Design review of the part shown in the three views and the two pictorial views. Dimensions are in mm from the part's minimum x, y and z. Round coordinates to 2 decimals unless told otherwise and drop trailing zeros. Loops run counter-clockwise (first coordinate to the right, second up) from the corner with the lowest first, then second, coordinate; pieces in that order, holes last. Notation, with made-up numbers: (77.5, -28.5) -> (130.5, -28.5) arc R21 ccw to (130.5, -6.5) -> close; hole circle Ø2 at (0, -31.75). An arc over 180 degrees is marked (long way). Write each question's results on one line, items separated by ' | '. Start each with the question number.
Item 1: We need section A-A (y = 22.5). Give the boundary of the cut face in (x, z) (3 decimals), and give its area (3 significant figures).
Item 2: Clearance check with flat-ended pins moving along their axes: pin 1 Ø10 at (x, y) = (51.5, 32) entering from -Z; pin 2 Ø8 at (x, y) = (35.875, 22.5) entering from +Z. State where each tip first meets the part, or that it passes through.
Item 3: We need section B-B (x = 37). Give the boundary of the cut face in (y, z).
Item 4: For L1, parallel to X at y = 22, z = 6.5; L2, parallel to Y at x = 37.5, z = 0.5; L3, parallel to Y at x = 130, z = 8.5, list the stretches that pass through material, from the lowest coordinate up. Write a range as from..to.
Item 5: We need section C-C (z = 2.5). Give the boundary of the cut face in (x, y) (3 decimals).
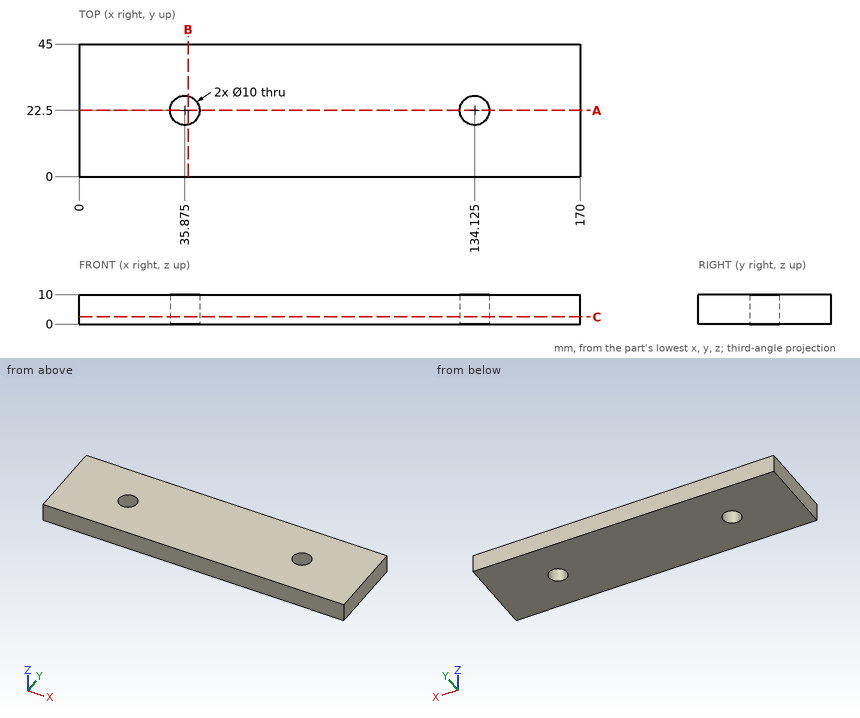
Here are the results:
1) outline: (0, 0) -> (30.875, 0) -> (30.875, 10) -> (0, 10) -> close; (40.875, 0) -> (129.125, 0) -> (129.125, 10) -> (40.875, 10) -> close; (139.125, 0) -> (170, 0) -> (170, 10) -> (139.125, 10) -> close | area: 1,500 mm2
2) pin 1: stops at z = 0 | pin 2: passes through
3) outline: (0, 0) -> (17.63, 0) -> (17.63, 10) -> (0, 10) -> close; (27.37, 0) -> (45, 0) -> (45, 10) -> (27.37, 10) -> close
4) L1: x = 0..30.9, 40.85..129.15, 139.1..170 | L2: y = 0..17.77, 27.23..45 | L3: y = 0..19.67, 25.33..45
5) outline: (0, 0) -> (170, 0) -> (170, 45) -> (0, 45) -> close; hole circle Ø10 at (35.875, 22.5); hole circle Ø10 at (134.125, 22.5)
